Can you work these out from the model? Positions are in its coordinate system, mm. A direction names the side the tool comes from. Round coordinates to 2 decimals unless told otherwise and drop trailing zeros. Order: outer loops, then holes, each group sorted by start corner. A loop starts at its lowest first (then second) coordinate and runs counter-clockwise, first axis right, second up. Notation, with made-up numbers: M 19,52.5 L 63,52.5 A20 cw 63,79.5 Z; hole C 5.25,89 d2. An arc over 180 degrees is marked long. Answer as a JSON object with one key per item and string values. Group by question number.
from build123d import *

# Parameters (mm, degrees)
F0_W     = 99.260524
F0_H     = 30.379737
F1_DEPTH = 9.144
F2_R     = 1.016
F3_R     = 1.597357
F3_R_2   = 1.808865
F3_R_3   = 1.82127
F3_R_4   = 1.741221
F4_DEPTH = 9.145
F3_R_5   = 9.801511
F3_R_6   = 5.336949
F5_DEPTH = 18.034


with BuildPart() as f1:
    # F0 (on Top) → F1 (new body)
    with BuildSketch(Plane.XY):
        with Locations((4.963025, -1.203157)):
            Rectangle(F0_W, F0_H)
    extrude(amount=F1_DEPTH)

    # F2
    f2_edges = [f1.edges().sort_by_distance(p)[0] for p in [
        (-44.667237, -1.203157, 9.144),
        (4.963025, 13.986711, 9.144),
        (4.963025, -16.393026, 9.144),
        (54.593287, -1.203157, 9.144),
        (54.593287, -1.203157, 0),
        (54.593287, 13.986711, 4.572),
        (54.593287, -16.393026, 4.572),
        (4.963025, 13.986711, 0),
        (-44.667237, 13.986711, 4.572),
        (-44.667237, -1.203157, 0),
        (-44.667237, -16.393026, 4.572),
        (4.963025, -16.393026, 0),
    ]]
    fillet(f2_edges, radius=F2_R)

    # F3 (on face) → F4 (cut, through all)
    with BuildSketch(Plane.XY.offset(9.144)):
        with Locations((50.720021, -12.913582)):
            Circle(F3_R)
        with Locations((50.474998, 9.873613)):
            Circle(F3_R_2)
        with Locations((-40.183738, 9.996125)):
            Circle(F3_R_3)
        with Locations((-40.673785, -12.423535)):
            Circle(F3_R_4)
    extrude(amount=-F4_DEPTH, mode=Mode.SUBTRACT)

    # F3 (on face) → F5 (join)
    with BuildSketch(Plane.XY.offset(9.144)):
        Circle(F3_R_5)
        Circle(F3_R_6, mode=Mode.SUBTRACT)
    extrude(amount=F5_DEPTH)


solid = f1.part
Item 1: Suppose I cut it at A-A, the plane x = 23. Write out the boundary of the cut face in (y, z), and give its area (3 significant figures).
Item 2: I'm going to push flat-ended pins straight in: pin 1 Ø3 at (x, y) = (50.72, -12.91) entering from -Z; pin 2 Ø5 at (y, z) = (11, 17) entering from +X; pin 3 Ø8 at (y, z) = (-10.5, 19) entering from +X; pin 4 Ø6 at (x, y) = (50.47, 9.87) entering from +Z. Where does each tip first touch, or does it pass through?
Item 3: On a 3-axis mill with a long thin cutter (end or side, diameter ignored), from which of +Z, -Z, +X, -X, +Y, -Y can I reach the whole of each face in a straight line? I mean faces 5 (the face through (4, 13.987, 5)), 6 (the face through (-0.695, 5.292, 18.035)). Say none if no direction works.
Item 4: I need wall thicknesses on line 1 (Z direction, x = 20, y = 12); line 2 (Y direction, x = -29, z = 8.25); line 3 (Y direction, x = 0, z = 23.25). Which ranges of each line are inside material? Lowest first, please.
Item 5: Suppose I cut it at D-D, the plane x = 0. Write out the boundary of the cut face in (y, z).
Item 6: Suppose I cut it at B-B, the plane z = 14. Write out the boundary of the cut face in (x, y), and give its area (3 significant figures).
Item 7: If we mould it in two halves opening along X, with no side actions, what happens to faces 1 (the face through (54.593, -1, 5)), 2 (the face through (4, -16.393, 5)), 3 (the face through (-38.447, 10.543, 4.636)), 4 (the face through (9.35, 2.94, 18.03))? For each: +X half, -X half, draft (parallel to the pull), parting line (faces both ways), or undercut.
Item 8: Suppose I cut it at C-C, the plane y = 0. Write out the boundary of the cut face in (x, z), and give its area (3 significant figures).
Computed:
{
 "1": {"outline": "M -16.39,1.02 A1.02 ccw -15.38,0 L 12.97,0 A1.02 ccw 13.99,1.02 L 13.99,8.13 A1.02 ccw 12.97,9.14 L -15.38,9.14 A1.02 ccw -16.39,8.13 Z", "area": "277 mm^2"},
 "2": {"pin 1": "passes through", "pin 2": "stops at x = 4.88", "pin 3": "stops at x = 7.34", "pin 4": "stops at z = 9.14"},
 "3": {"face 5": "+Z, -Z, +X, -X, +Y", "face 6": "+Z"},
 "4": {"line 1": "z = 0 to 9.14", "line 2": "y = -16.39 to 13.98", "line 3": "y = -9.8 to -5.34, 5.34 to 9.8"},
 "5": {"outline": "M -16.39,1.02 A1.02 ccw -15.38,0 L 12.97,0 A1.02 ccw 13.99,1.02 L 13.99,8.13 A1.02 ccw 12.97,9.14 L 9.8,9.14 L 9.8,27.18 L 5.34,27.18 L 5.34,9.14 L -5.34,9.14 L -5.34,27.18 L -9.8,27.18 L -9.8,9.14 L -15.38,9.14 A1.02 ccw -16.39,8.13 Z"},
 "6": {"outline": "C 0,0 d19.6; hole C 0,0 d10.67", "area": "212 mm^2"},
 "7": {"face 1": "+X half", "face 2": "draft", "face 3": "undercut", "face 4": "parting line"},
 "8": {"outline": "M -44.67,1.02 A1.02 ccw -43.65,0 L 53.58,0 A1.02 ccw 54.59,1.02 L 54.59,8.13 A1.02 ccw 53.58,9.14 L 9.8,9.14 L 9.8,27.18 L 5.34,27.18 L 5.34,9.14 L -5.34,9.14 L -5.34,27.18 L -9.8,27.18 L -9.8,9.14 L -43.65,9.14 A1.02 ccw -44.67,8.13 Z", "area": "1,070 mm^2"}
}
